Can you work these out from the model? Positions are in its coordinate system, mm. Face numbers are marked on the shaded views. A direction names the side the tool comes from. Give positions to 0.01 mm unless a question says otherwise; leave off trailing zeros. Order: outer loops, then holes, each group sorted by start corner. A loop starts at its lowest first (then second) coordinate and runs counter-clockwise, first axis right, second up. Notation, with made-up numbers: (48.25, -39.5) -> (76.25, -39.5) arc R14 ccw to (76.25, -33.5) -> close; hole circle Ø9 at (85.5, 32). An arc over 180 degrees is marked (long way). Answer as a JSON object with one key per item and string values.
```python
from build123d import *

# Parameters (mm, degrees)
EXTRUDE_1_DEPTH     = 170
SHELL_7_T           = -4
CUT_EXTRUDE_2_DEPTH = 2
CUT_EXTRUDE_4_DEPTH = 162
CHAMFER_2_SIZE      = 3.6
SKETCH_7_R          = 2.4
CUT_EXTRUDE_5_DEPTH = 10


with BuildPart() as part:
    # 草图1 → 凸台-拉伸1 (new body)
    with BuildSketch(Plane.XY):
        Polygon((0, 0), (0, -21.28355545), (-28.190778624, -11.02295115), (-97.922791811, 138.517833711), (-79.79663607, 146.970198946), (-13.565707197, 4.937513627), align=None)
    extrude(amount=EXTRUDE_1_DEPTH)

    # 抽壳7
    shell_7_openings = [part.faces().sort_by_distance(p)[0] for p in [
        (0, -10.641777725, 85),
        (-6.782853599, 2.468756813, 85),
        (-46.681171634, 75.953856286, 85),
        (-88.85971394, 142.744016329, 85),
    ]]
    offset(amount=SHELL_7_T, openings=shell_7_openings, kind=Kind.INTERSECTION)

    # 草图4 → 切除-拉伸2 (cut)
    with BuildSketch(Plane.XY.offset(170)):
        with BuildLine():
            Line((-81.234877122, 135.26575694), (-78.593512986, 129.601333271))
            Line((-78.593512986, 129.601333271), (-85.390821389, 126.431696308))
            Line((-85.390821389, 126.431696308), (-88.032185524, 132.096119977))
            ThreePointArc((-88.032185524, 132.096119977), (-86.218349805, 137.07959266), (-81.234877122, 135.26575694))
        make_face()
    extrude(amount=-CUT_EXTRUDE_2_DEPTH, mode=Mode.SUBTRACT)

    # 草图2 → 切除-拉伸4 (cut)
    with BuildSketch(Plane.XY.offset(4)):
        Polygon((0, -20.88355545), (-19.529222148, -9.608353785), (0, -9.608353785), align=None)
    extrude(amount=CUT_EXTRUDE_4_DEPTH, mode=Mode.SUBTRACT)

    # 倒角2
    chamfer_2_edges = [part.edges().sort_by_distance(p)[0] for p in [
        (0, -10.441777725, 166),
        (0, -10.441777725, 4),
    ]]
    chamfer(chamfer_2_edges, length=CHAMFER_2_SIZE)

    # 草图7 → 切除-拉伸5 (cut)
    with BuildSketch(Plane(origin=(0, 0, 0), x_dir=(-1, 0, 0), z_dir=(0, 0, -1))):
        with Locations((84.633531323, 133.680938458)):
            Circle(SKETCH_7_R)
    extrude(amount=-CUT_EXTRUDE_5_DEPTH, mode=Mode.SUBTRACT)


solid = part.part
```
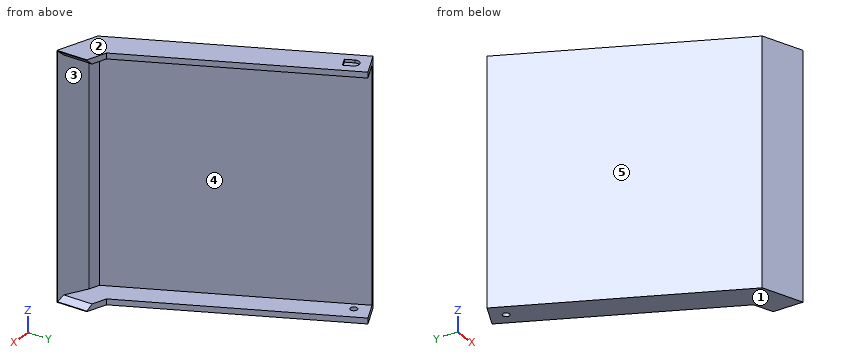
1. If we mould it in two halves opening along Z, with no side actions, what happens to the marked faces 1, 2 and 3? For each: +Z half, -Z half, draft (parallel to the pull), parting line (faces both ways), or undercut.
Worked answers:
{"face 1": "-Z half", "face 2": "+Z half", "face 3": "undercut"}
2. Will these pins go through, and if not, where does the flat tip stop? pin 1 Ø5 at (x, y) = (-81.5, 133) entering from +Z; pin 2 Ø3 at (x, z) = (-42, 34) entering from +Y; pin 3 Ø6 at (x, z) = (-21.5, 132) entering from +Y; pin 4 Ø8 at (x, z) = (-28.5, 19) entering from -Y.
Worked answers:
{"pin 1": "z = 170", "pin 2": "y = 31.27", "pin 3": "y = -8.11", "pin 4": "y = -12.37"}
3. Please list where these lines run through material, in increasing order: L1, parallel to Z at x = -35.5, y = 37; L2, parallel to Y at x = -66, z = 50.5; L3, parallel to X at y = -7.5, z = 76.
Worked answers:
{"L1": "0 to 4, 166 to 170", "L2": "70.06 to 79.52", "L3": "-29.83 to -25.42"}
4. If we section it at C-C on y = 18: Please give me the cut outline in (x, z), then the cut area to 3 significant figures.
Worked answers:
{"outline": "(-41.72, 0) -> (-19.66, 0) -> (-19.66, 4) -> (-37.31, 4) -> (-37.31, 166) -> (-19.66, 166) -> (-19.66, 170) -> (-41.72, 170) -> close", "area": "892 mm²"}
5. If we section it at B-B on x = -64: Please give me the cut outline in (y, z), then the cut area to 3 significant figures.
Worked answers:
{"outline": "(65.77, 0) -> (113.09, 0) -> (113.09, 4) -> (75.23, 4) -> (75.23, 166) -> (113.09, 166) -> (113.09, 170) -> (65.77, 170) -> close", "area": "1,910 mm²"}
6. For the marked faces 4 and 5, which set-ups out of +Z, -Z, +X, -X, +Y, -Y let a thin tool reach every point of the face, with its end or its side?
Worked answers:
{"face 4": "+X, +Y", "face 5": "+Z, -Z, -X, -Y"}
7. If we section it at A-A on z = 29.5: Please give me the cut outline in (x, y).
Worked answers:
{"outline": "(-97.92, 138.52) -> (-28.19, -11.02) -> (0, -21.28) -> (0, -20.88) -> (-18.07, -10.45) -> (-25.27, -7.83) -> (-94.3, 140.21) -> close"}
